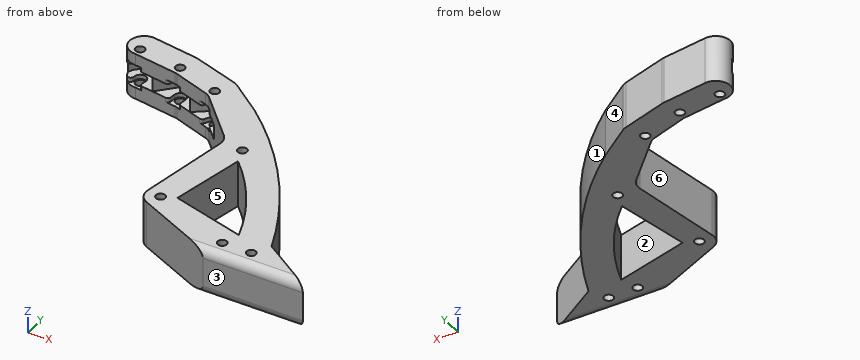
```python
from build123d import *

# Parameters (mm, degrees)
SKETCH1_R           = 1.6
BOSS_EXTRUDE1_DEPTH = 16
FILLET1_R           = 3
FILLET2_R           = 5
CUT_EXTRUDE1_START  = -5.5
SKETCH2_R           = 2.1
SKETCH2_R_2         = 1.6
CUT_EXTRUDE1_DEPTH  = 5
CUT_EXTRUDE2_START  = -4
SKETCH2_4_R         = 1.6
CUT_EXTRUDE2_DEPTH  = 8
FILLET3_R           = 1


with BuildPart() as part:
    # Sketch1 → Boss-Extrude1 (new body)
    with BuildSketch(Plane.XY):
        with BuildLine():
            Line((59.46, -17), (41.32, -5))
            ThreePointArc((41.32, -5), (24.459745553, 26.441207242), (0.2, 52.6))
            Line((0.2, 52.6), (-11, 61))
            ThreePointArc((-11, 61), (-11.709245402, 61.444372101), (-12.482677345, 61.764213677))
            Line((-12.482677345, 61.764213677), (-27.982677345, 66.70070535))
            Line((-27.982677345, 66.70070535), (-28.761883628, 66.881709992))
            Line((-28.761883628, 66.881709992), (-44.261883628, 69.195218319))
            ThreePointArc((-44.261883628, 69.195218319), (-49.986285772, 64.62007324), (-45, 59.25))
            Line((-45, 59.25), (-29.5, 56.936491673))
            Line((-29.5, 56.936491673), (-15.593484906, 52.260716736))
            Line((-15.593484906, 52.260716736), (1, 35))
            Line((1, 35), (-4.926348457, 0.855038527))
            ThreePointArc((-4.926348457, 0.855038527), (-4.425801292, -2.326431372), (-2.089024899, -4.542683675))
            Line((-2.089024899, -4.542683675), (25, -17))
            Line((25, -17), (59.46, -17))
        make_face()
        with Locations((28, -11)):
            Circle(SKETCH1_R, mode=Mode.SUBTRACT)
        with Locations((38, -11)):
            Circle(SKETCH1_R, mode=Mode.SUBTRACT)
        with BuildLine():
            Line((30.019916022, -5), (4.581128304, 2.00331312))
            Line((4.581128304, 2.00331312), (9.851129428, 27.519340358))
            ThreePointArc((9.851129428, 27.519340358), (21.90850327, 12.483330411), (30.019916022, -5))
        make_face(mode=Mode.SUBTRACT)
        with Locations((-45, 62)):
            Circle(SKETCH1_R, mode=Mode.SUBTRACT)
        with Locations((-30, 60)):
            Circle(SKETCH1_R, mode=Mode.SUBTRACT)
        with Locations((-15, 55)):
            Circle(SKETCH1_R, mode=Mode.SUBTRACT)
        with Locations((8, 33)):
            Circle(SKETCH1_R, mode=Mode.SUBTRACT)
        Circle(SKETCH1_R, mode=Mode.SUBTRACT)
    extrude(amount=BOSS_EXTRUDE1_DEPTH)

    # Fillet1
    fillet1_edges = [part.edges().sort_by_distance(p)[0] for p in [
        (42.23, -17, 0),
        (42.23, -17, 16),
    ]]
    fillet(fillet1_edges, radius=FILLET1_R)

    # Fillet2
    fillet2_edges = [part.edges().sort_by_distance(p)[0] for p in [
        (1, 35, 8),
        (-15.593484906, 52.260716736, 8),
        (-29.5, 56.936491673, 8),
    ]]
    fillet(fillet2_edges, radius=FILLET2_R)

    # Sketch2 → Cut-Extrude1 (cut)
    # profile 1 of 3: a face of its own
    with BuildSketch(Plane.XY.offset(16).offset(CUT_EXTRUDE1_START)):
        with BuildLine():
            Line((-23.499613929, 54.918987315), (-16.755150829, 52.651302614))
            ThreePointArc((-16.755150829, 52.651302614), (-15.672698928, 52.135686265), (-14.744120066, 51.377198536))
            Line((-14.744120066, 51.377198536), (-10, 46.442315172))
            Line((-10, 46.442315172), (-10, 55))
            ThreePointArc((-10, 55), (-12.752546223, 59.466424915), (-17.979580608, 59.015233418))
            Line((-17.979580608, 59.015233418), (-23.499613929, 54.918987315))
        make_face()
        with Locations((-15, 55)):
            Circle(SKETCH2_R, mode=Mode.SUBTRACT)
    # profile 2 of 3: a face of its own
    with BuildSketch(Plane.XY.offset(16).offset(CUT_EXTRUDE1_START)):
        with BuildLine():
            Line((-23.499613929, 54.918987315), (-25.163326304, 61.267512349))
            ThreePointArc((-25.163326304, 61.267512349), (-28.762198184, 64.844362359), (-33.635794756, 63.432345625))
            Line((-33.635794756, 63.432345625), (-38.5, 58.279819089))
            Line((-38.5, 58.279819089), (-29.936778714, 57.001684653))
            ThreePointArc((-29.936778714, 57.001684653), (-29.504556057, 56.917567707), (-29.081410179, 56.795749598))
            Line((-29.081410179, 56.795749598), (-23.499613929, 54.918987315))
        make_face()
        with Locations((-30, 60)):
            Circle(SKETCH2_R_2, mode=Mode.SUBTRACT)
    # profile 3 of 3: a face of its own
    with BuildSketch(Plane.XY.offset(16).offset(CUT_EXTRUDE1_START)):
        with BuildLine():
            Line((-38.5, 58.279819089), (-40.253762465, 63.572650394))
            ThreePointArc((-40.253762465, 63.572650394), (-45.2324625, 66.994593195), (-49.871793817, 63.125))
            ThreePointArc((-49.871793817, 63.125), (-48.112474899, 60.336881039), (-45, 59.25))
            Line((-45, 59.25), (-38.5, 58.279819089))
        make_face()
        with Locations((-45, 62)):
            Circle(SKETCH2_R, mode=Mode.SUBTRACT)
    extrude(amount=-CUT_EXTRUDE1_DEPTH, mode=Mode.SUBTRACT)

    # Sketch2<4> → Cut-Extrude2 (cut)
    # profile 1 of 3: a face of its own
    with BuildSketch(Plane.XY.offset(16).offset(CUT_EXTRUDE2_START)):
        with BuildLine():
            Line((-16.799757531, 56.082068773), (-18.50808127, 53.240688824))
            Line((-18.50808127, 53.240688824), (-16.755150829, 52.651302614))
            ThreePointArc((-16.755150829, 52.651302614), (-15.672698928, 52.135686265), (-14.744120066, 51.377198536))
            Line((-14.744120066, 51.377198536), (-13.205359072, 53.909466214))
            ThreePointArc((-13.205359072, 53.909466214), (-13.913695708, 56.797204214), (-16.799757531, 56.082068773))
        make_face()
        with Locations((-15, 55)):
            Circle(SKETCH2_4_R, mode=Mode.SUBTRACT)
    # profile 2 of 3: a face of its own
    with BuildSketch(Plane.XY.offset(16).offset(CUT_EXTRUDE2_START)):
        with BuildLine():
            Line((-29.081410179, 56.795749598), (-28.352112311, 56.550538438))
            Line((-28.352112311, 56.550538438), (-27.919359393, 59.715509815))
            ThreePointArc((-27.919359393, 59.715509815), (-29.718455545, 62.081041259), (-32.08143774, 60.27859816))
            Line((-32.08143774, 60.27859816), (-32.469451039, 57.379707783))
            Line((-32.469451039, 57.379707783), (-29.936778714, 57.001684653))
            ThreePointArc((-29.936778714, 57.001684653), (-29.504556057, 56.917567707), (-29.081410179, 56.795749598))
        make_face()
        with Locations((-30, 60)):
            Circle(SKETCH2_4_R, mode=Mode.SUBTRACT)
    # profile 3 of 3: a face of its own
    with BuildSketch(Plane.XY.offset(16).offset(CUT_EXTRUDE2_START)):
        with BuildLine():
            Line((-45, 59.25), (-43.396661475, 59.010687934))
            Line((-43.396661475, 59.010687934), (-42.932168542, 61.633840116))
            ThreePointArc((-42.932168542, 61.633840116), (-44.635424811, 64.068111441), (-47.068390209, 62.36299028))
            Line((-47.068390209, 62.36299028), (-47.497405572, 59.918376123))
            ThreePointArc((-47.497405572, 59.918376123), (-46.292648563, 59.419983469), (-45, 59.25))
        make_face()
        with Locations((-45, 62)):
            Circle(SKETCH2_4_R, mode=Mode.SUBTRACT)
    extrude(amount=-CUT_EXTRUDE2_DEPTH, mode=Mode.SUBTRACT)

    # Fillet3
    fillet3_edges = [part.edges().sort_by_distance(p)[0] for p in [
        (-14.744120066, 51.377198536, 4.75),
        (-14.744120066, 51.377198536, 11.25),
        (-18.50808127, 53.240688824, 11.25),
        (-18.50808127, 53.240688824, 4.75),
        (-43.396661475, 59.010687934, 11.25),
        (-47.497405572, 59.918376123, 11.25),
        (-43.396661475, 59.010687934, 4.75),
        (-47.497405572, 59.918376123, 4.75),
        (-28.352112311, 56.550538438, 11.25),
        (-32.469451039, 57.379707783, 11.25),
        (-28.352112311, 56.550538438, 4.75),
        (-32.469451039, 57.379707783, 4.75),
    ]]
    fillet(fillet3_edges, radius=FILLET3_R)


solid = part.part
```
The listing builds one solid part. Answer for the finished solid, in the listing's coordinates (mm). Face numbers are marked on the shaded views. A direction names the side the tool comes from. Coordinates: 2 decimals unless noted, no trailing zeros. Write each loop counter-clockwise with the first axis right and the second up, starting at its lowest first coordinate (ties: lowest second). Pieces come first, ordered by that corner, then holes. Notation, with made-up numbers: M 30.5,23 L 50.5,23 A8 cw 50.5,32 Z; hole C 68.5,5 d6. An arc over 180 degrees is marked long. Use a Markdown table: item, result. Add a question column.
1. Section A-A (z = 7.5) is taken. Count the separate pieces of the cut face and the enclosed holes in it, plus the area to 3 significant figures.
2. Section C-C (x = 28) is taken. Give the vertices of the cut face in (y, z).
3. Section D-D (x = -22) is taken. Give the vertices of the cut face in (y, z).
4. For a pull along Y with two mould halves and no side action, classify the marked faces 3, 4, 5 and 6 as +Y half, -Y half, draft (parallel to the pull), parting line (faces both ways), or undercut.
5. Which of the six approach directions +Z, -Z, +X, -X, +Y, -Y give full straight-line access (tool end or side, diameter ignored) to the marked faces 1 and 2?
6. Given P1, Ø4, axis at x = -38.5, z = 6.5, coming from the +Y side; P2, Ø5, axis at x = -18.5, z = 12, coming from the -Y side; P3, Ø1, axis at x = -29, z = 7, coming from the -Y side, each flat-ended and moving along its own axis, determine where each tip first touches the part or whether it passes through.
7. Section B-B (y = 10) is taken. Give the vertices of the cut face in (x, z).
8. Straight lines are drawn through the part: line 1 along Y through (x, z) = (-45, 2.95); line 2 along Y through (x, z) = (20, 6.5); line 3 along X through (y, z) = (10, 4.75). For each, find the intervals that lie inside material, in ascending order. Write a range as [from, to].
Data:
| question | item | result |
|---|---|---|
| 1 | separate pieces | 1 |
| 1 | enclosed holes | 5 |
| 1 | area | 1,850 mm2 |
| 2 | outline | M -17,3 A3 ccw -14,0 L -12.6,0 L -12.6,16 L -14,16 A3 ccw -17,13 Z; M -9.4,0 L -4.44,0 L -4.44,16 L -9.4,16 Z; M 0.53,0 L 21.24,0 L 21.24,16 L 0.53,16 Z |
| 3 | outline | M 54.41,0 L 64.8,0 L 64.8,16 L 54.41,16 L 54.41,10.5 L 56.03,10.5 L 56.03,5.5 L 54.41,5.5 Z |
| 4 | face 3 | -Y half |
| 4 | face 4 | +Y half |
| 4 | face 5 | undercut |
| 4 | face 6 | undercut |
| 5 | face 1 | +Z, -Z, +X, +Y |
| 5 | face 2 | +Z, -Z |
| 6 | P1 | stops at y = 68.63 |
| 6 | P2 | stops at y = 52.33 |
| 6 | P3 | stops at y = 64.77 |
| 7 | outline | M -3.34,0 L 6.23,0 L 6.23,16 L -3.34,16 Z; M 23.39,0 L 34.56,0 L 34.56,16 L 23.39,16 Z |
| 8 | line 1 | y = [59.25, 60.4], [63.6, 69.25] |
| 8 | line 2 | y = [-14.7, -2.24], [15.42, 32.35] |
| 8 | line 3 | x = [-3.34, 6.23], [23.39, 34.56] |
